Could you check a few things on this model? Use its own coordinates, in mm. A direction names the side the tool comes from. Coordinates: 2 decimals unless noted, no trailing zeros. Loops run counter-clockwise (first coordinate to the right, second up) from the corner with the lowest first, then second, coordinate; pieces in that order, holes last.
from build123d import *

# Parameters (mm, degrees)
ESTRUSIONE_ESTRUSIONE1_DEPTH  = 10
TAGLIO_ESTRUSIONE1_DEPTH      = 3
SCHIZZO4_W                    = 80
SCHIZZO4_H                    = 5
ESTRUSIONE_ESTRUSIONE2_DEPTH  = 35
ESTRUSIONE_ESTRUSIONE4_DEPTH  = 80
SCHIZZO7_W                    = 80
SCHIZZO7_H                    = 5
ESTRUSIONE_ESTRUSIONE5_DEPTH  = 7
TAGLIO_ESTRUSIONE2_REACH      = 42
SCHIZZO8_R                    = 1.5
RACCORDO1_R                   = 5
RACCORDO2_R                   = 5
TAGLIO_ESTRUSIONE3_DEPTH      = 1
TAGLIO_ESTRUSIONE3_DEPTH_BACK = 10
SCHIZZO11_R                   = 4
TAGLIO_ESTRUSIONE4_DEPTH      = 3
SCHIZZO12_W                   = 12
SCHIZZO12_H                   = 12
ESTRUSIONE_ESTRUSIONE6_DEPTH  = 40
SCHIZZO13_R                   = 1.5
TAGLIO_ESTRUSIONE5_DEPTH      = 41
SCHIZZO14_R                   = 4
TAGLIO_ESTRUSIONE6_DEPTH      = 10


with BuildPart() as part:
    # Schizzo1 → Estrusione-Estrusione1 (new body)
    with BuildSketch(Plane.XY):
        with BuildLine():
            Line((-76.016095604, 20), (76.016095604, 20))
            ThreePointArc((76.016095604, 20), (92.5, 0), (76.016095604, -20))
            Line((76.016095604, -20), (-76.016095604, -20))
            ThreePointArc((-76.016095604, -20), (-92.5, 0), (-76.016095604, 20))
        make_face()
    extrude(amount=ESTRUSIONE_ESTRUSIONE1_DEPTH)

    # Schizzo3 → Taglio-Estrusione1 (cut)
    with BuildSketch(Plane.XY.offset(10)):
        with BuildLine():
            Line((-75.5, -15), (75.5, -15))
            ThreePointArc((75.5, -15), (87.5, 0), (75.5, 15))
            Line((75.5, 15), (-75.5, 15))
            ThreePointArc((-75.5, 15), (-87.5, 0), (-75.5, -15))
        make_face()
    extrude(amount=-TAGLIO_ESTRUSIONE1_DEPTH, mode=Mode.SUBTRACT)

    # Schizzo4 → Estrusione-Estrusione2 (add)
    with BuildSketch(Plane.XY.offset(10)):
        with Locations((0, -17.5)):
            Rectangle(SCHIZZO4_W, SCHIZZO4_H)
    estrusione_estrusione2 = extrude(amount=ESTRUSIONE_ESTRUSIONE2_DEPTH)

    # Schizzo6 → Estrusione-Estrusione4 (add)
    with BuildSketch(Plane(origin=(40, 0, 0), x_dir=(0, 0, -1), z_dir=(1, 0, 0))):
        Polygon((-40, -15), (-40, -12.81), (-7, -15), align=None)
    estrusione_estrusione4 = extrude(amount=-ESTRUSIONE_ESTRUSIONE4_DEPTH)

    # Schizzo7 → Estrusione-Estrusione5 (add)
    with BuildSketch(Plane(origin=(0, -15, 0), x_dir=(1, 0, 0), z_dir=(0, 1, 0))):
        with Locations((0, -42.5)):
            Rectangle(SCHIZZO7_W, SCHIZZO7_H)
    estrusione_estrusione5 = extrude(amount=ESTRUSIONE_ESTRUSIONE5_DEPTH)

    # Schizzo8 → Taglio-Estrusione2 (cut, up to next)
    with BuildSketch(Plane.XZ.offset(20), mode=Mode.PRIVATE) as taglio_estrusione2_sk1:
        with Locations((-30, 13)):
            Circle(SCHIZZO8_R)
    taglio_estrusione2_tool1 = extrude(taglio_estrusione2_sk1.sketch, amount=-TAGLIO_ESTRUSIONE2_REACH, mode=Mode.PRIVATE) & part.part
    add(taglio_estrusione2_tool1.solids().sort_by_distance((-30, -20, 13))[0], mode=Mode.SUBTRACT)
    # Schizzo8 → Taglio-Estrusione2 (cut, up to next)
    with BuildSketch(Plane.XZ.offset(20), mode=Mode.PRIVATE) as taglio_estrusione2_sk2:
        with Locations((-30, 32)):
            Circle(SCHIZZO8_R)
    taglio_estrusione2_tool2 = extrude(taglio_estrusione2_sk2.sketch, amount=-TAGLIO_ESTRUSIONE2_REACH, mode=Mode.PRIVATE) & part.part
    add(taglio_estrusione2_tool2.solids().sort_by_distance((-30, -20, 32))[0], mode=Mode.SUBTRACT)
    # Schizzo8 → Taglio-Estrusione2 (cut, up to next)
    with BuildSketch(Plane.XZ.offset(20), mode=Mode.PRIVATE) as taglio_estrusione2_sk3:
        with Locations((30, 13)):
            Circle(SCHIZZO8_R)
    taglio_estrusione2_tool3 = extrude(taglio_estrusione2_sk3.sketch, amount=-TAGLIO_ESTRUSIONE2_REACH, mode=Mode.PRIVATE) & part.part
    add(taglio_estrusione2_tool3.solids().sort_by_distance((30, -20, 13))[0], mode=Mode.SUBTRACT)
    # Schizzo8 → Taglio-Estrusione2 (cut, up to next)
    with BuildSketch(Plane.XZ.offset(20), mode=Mode.PRIVATE) as taglio_estrusione2_sk4:
        with Locations((30, 32)):
            Circle(SCHIZZO8_R)
    taglio_estrusione2_tool4 = extrude(taglio_estrusione2_sk4.sketch, amount=-TAGLIO_ESTRUSIONE2_REACH, mode=Mode.PRIVATE) & part.part
    add(taglio_estrusione2_tool4.solids().sort_by_distance((30, -20, 32))[0], mode=Mode.SUBTRACT)

    # Specchia1: Estrusione-Estrusione2, Estrusione-Estrusione4, Estrusione-Estrusione5 across plane
    add(estrusione_estrusione2.mirror(Plane.ZX))
    add(estrusione_estrusione4.mirror(Plane.ZX))
    add(estrusione_estrusione5.mirror(Plane.ZX))

    # Raccordo1
    raccordo1_edges = [part.edges().sort_by_distance(p)[0] for p in [
        (0, -20, 45),
    ]]
    fillet(raccordo1_edges, radius=RACCORDO1_R)

    # Raccordo2
    raccordo2_edges = [part.edges().sort_by_distance(p)[0] for p in [
        (0, 20, 45),
    ]]
    fillet(raccordo2_edges, radius=RACCORDO2_R)

    # Schizzo9 → Taglio-Estrusione3 (cut, two sides)
    with BuildSketch(Plane.XZ.offset(20)) as taglio_estrusione3_sk:
        Polygon((-4, 11), (-4, 3), (4, 3), (4, 11), (10, 11), (10, 31), (-10, 31), (-10, 11), align=None)
    extrude(amount=TAGLIO_ESTRUSIONE3_DEPTH, mode=Mode.SUBTRACT)
    extrude(taglio_estrusione3_sk.sketch, amount=-TAGLIO_ESTRUSIONE3_DEPTH_BACK, mode=Mode.SUBTRACT)

    # Schizzo11 → Taglio-Estrusione4 (cut)
    with BuildSketch(Plane(origin=(0, -15.396736192, 1.021783402), x_dir=(1, 0, 0), z_dir=(0, 0.997805181, -0.06621798))):
        with Locations((-30, -12.004564445)):
            Circle(SCHIZZO11_R)
        with Locations((-30, -31.046357736)):
            Circle(SCHIZZO11_R)
        with Locations((30, -31.046357736)):
            Circle(SCHIZZO11_R)
        with Locations((30, -12.004564445)):
            Circle(SCHIZZO11_R)
    extrude(amount=-TAGLIO_ESTRUSIONE4_DEPTH, mode=Mode.SUBTRACT)

    # Schizzo12 → Estrusione-Estrusione6 (add)
    with BuildSketch(Plane.XZ.offset(20)):
        with Locations((70.016095604, -6)):
            Rectangle(SCHIZZO12_W, SCHIZZO12_H)
        with Locations((-70.016095604, -6)):
            Rectangle(SCHIZZO12_W, SCHIZZO12_H)
        with Locations((0, -6)):
            Rectangle(SCHIZZO12_W, SCHIZZO12_H)
    extrude(amount=-ESTRUSIONE_ESTRUSIONE6_DEPTH)

    # Schizzo13 → Taglio-Estrusione5 (cut, through all)
    with BuildSketch(Plane.XZ.offset(20)):
        with Locations((-70.016095604, -6)):
            Circle(SCHIZZO13_R)
        with Locations((0, -6)):
            Circle(SCHIZZO13_R)
        with Locations((70.016095604, -6)):
            Circle(SCHIZZO13_R)
    extrude(amount=-TAGLIO_ESTRUSIONE5_DEPTH, mode=Mode.SUBTRACT)

    # Schizzo14 → Taglio-Estrusione6 (cut)
    with BuildSketch(Plane.XZ.offset(20)):
        with Locations((-70.016095604, -6)):
            Circle(SCHIZZO14_R)
        with Locations((0, -6)):
            Circle(SCHIZZO14_R)
        with Locations((70.016095604, -6)):
            Circle(SCHIZZO14_R)
    taglio_estrusione6 = extrude(amount=-TAGLIO_ESTRUSIONE6_DEPTH, mode=Mode.SUBTRACT)

    # Specchia2: Taglio-Estrusione6 across plane
    add(taglio_estrusione6.mirror(Plane.ZX), mode=Mode.SUBTRACT)


solid = part.part
(1) Imagine slicing it at D-D, the plane y = 3. Write out the boundary of the cut face in (x, z), and give its area (3 significant figures).
Answers:
outline: (-92.28, 0) - (-76.02, 0) - (-76.02, -12) - (-64.02, -12) - (-64.02, 0) - (-6, 0) - (-6, -12) - (6, -12) - (6, 0) - (64.02, 0) - (64.02, -12) - (76.02, -12) - (76.02, 0) - (92.28, 0) - (92.28, 10) - (87.2, 10) - (87.2, 7) - (-87.2, 7) - (-87.2, 10) - (-92.28, 10) - close; hole circle Ø3 at (-70.02, -6); hole circle Ø3 at (0, -6); hole circle Ø3 at (70.02, -6)
area: 1,730 mm2
(2) For pin 1 (9 mm diameter, centred on y = -15, z = 5.5, fed in from -X); pin 2 (3 mm diameter, centred on x = -55, y = 4.5, fed in from -Z); pin 3 (4 mm diameter, centred on x = -71.5, z = -7, fed in from -Y), each with a flat end and sliding along its axis, tell me the tip position at first contact or that it passes through.
Answers:
pin 1: stops at x = -89.59
pin 2: stops at z = 0
pin 3: stops at y = -10
(3) I need wall thicknesses on probe 1 along X at (y, z) = (-15, -0.5); probe 2 along Z at (x, y) = (0, -12); probe 3 along Z at (x, y) = (30, -19). Which ranges of each line are inside material? Lowest first, please.
Answers:
probe 1: x = -76.02 to -64.02, -6 to 6, 64.02 to 76.02
probe 2: z = -12 to -10, -2 to 3, 40 to 45
probe 3: z = 0 to 11.5, 14.5 to 30.5, 33.5 to 43
(4) Imagine slicing it at A-A, the plane z = 25. Write out the boundary of the cut face in (x, y).
Answers:
outline: (-40, -20) - (-10, -20) - (-10, -13.81) - (-40, -13.81) - close; (-40, 13.81) - (40, 13.81) - (40, 20) - (-40, 20) - close; (10, -20) - (40, -20) - (40, -13.81) - (10, -13.81) - close
(5) Which directions (+Z, -Z, +X, -X, +Y, -Y) give clear straight access to the entire face, cutting with the end or side of a thin tool? Please do faces 1 (the face through (-82, 0, 0)), 2 (the face through (-28.3, -17.6, 13.1)), 3 (the face through (-35, 0, 0)), 4 (the face through (58, -15, 9)), 5 (the face through (-70, 10, -8)).
Answers:
face 1: -Z, -X, +Y, -Y
face 2: none
face 3: -Z, +Y, -Y
face 4: +Z
face 5: +Y
(6) We'd pull the mould along Y, two halves only. Please class faces 6 (the face through (68.826, -0.14, -6.913)), 7 (the face through (92.496, 0.393, 4.93)), 8 (the face through (58, 15, 9)), 9 (the face through (-1, 10, 40)): +Y half, -Y half, draft (parallel to the pull), parting line (faces both ways), or undercut.
Answers:
face 6: draft
face 7: parting line
face 8: undercut
face 9: undercut
(7) Imagine slicing it at B-B, the plane y = -5. Write out the boundary of the cut face in (x, z).
Answers:
outline: (-91.88, 0) - (-76.02, 0) - (-76.02, -12) - (-64.02, -12) - (-64.02, 0) - (-6, 0) - (-6, -12) - (6, -12) - (6, 0) - (64.02, 0) - (64.02, -12) - (76.02, -12) - (76.02, 0) - (91.88, 0) - (91.88, 10) - (86.66, 10) - (86.66, 7) - (-86.66, 7) - (-86.66, 10) - (-91.88, 10) - close; hole circle Ø3 at (-70.02, -6); hole circle Ø3 at (0, -6); hole circle Ø3 at (70.02, -6)
(8) Imagine slicing it at C-C, the plane x = -44.5. Write out the boundary of the cut face in (y, z).
Answers:
outline: (-20, 0) - (20, 0) - (20, 10) - (15, 10) - (15, 7) - (-15, 7) - (-15, 10) - (-20, 10) - close
